The listing builds one solid part. Answer for the finished solid, in the listing's coordinates (mm). A direction names the side the tool comes from. Coordinates: 2 decimals unless noted, no trailing zeros. Order: outer loops, then holes, each group sorted by start corner. A loop starts at its lowest first (then second) coordinate and runs counter-clockwise, first axis right, second up. Notation, with made-up numbers: (-27, 45) - (-20, 45) arc R16 ccw to (-20, 72) - close; hole circle Ø10 at (76, 63.5). An arc over 180 degrees is marked (long way). Use a Markdown table: item, result. Add a question column.
Item 1: Flat-ended cylindrical pins translate along their axes: P1, Ø2, axis at x = -5.5, y = 15, coming from the +Z side; P2, Ø9, axis at x = -1, z = -9, coming from the +Y side; P3, Ø2.5, axis at x = -2, y = 14, coming from the +Z side. Find the tip coordinate at first contact, or state that the pin passes through.
Item 2: The part is cut by section D-D, the plane x = 6.25. Give the vertices of the cut face in (y, z), then the cut area to 3 significant figures.
Item 3: The mould has two halves that part along X. Classify faces 5 (the cylindrical face through (0.358, 17.477, -26.105)), 6 (the flat face through (0, 4, 0)), 7 (the cylindrical face through (0.596, 3.882, -4.815)), 8 (the flat face through (-6, 12.1, -28.2)): released by +X, released by -X, zero draft, split by the parting line, or undercut.
Item 4: The part is cut by section A-A, the plane x = 0. Give the vertices of the cut face in (y, z) (3 decimals).
Item 5: For faces 1 (the flat face through (0.9, 7.9, -10.4)), 2 (the flat face through (-6.1, 1.9, -7.6)), 3 (the flat face through (-6, 4, -15.5)), 4 (the flat face through (-6, 5.75, -8)), determine the directions among +Z, -Z, +X, -X, +Y, -Y from which every point of the face is accessible in a straight line to the end or side of a thin tool.
Item 6: Find the intervals of material crossed by line 1 along Z through (x, y) = (0, 3.5); line 2 along Y through (x, z) = (-6, -27.75); line 3 along Z through (x, y) = (-2.5, 18), in increasing order.
Item 7: The part is cut by section B-B, the plane y = 14.75. Give the vertices of the cut face in (x, z).
Item 8: The part is cut by section C-C, the plane z = -7.5. Give the vertices of the cut face in (x, y) (3 decimals).
from build123d import *

# Parameters (mm, degrees)
ESTRUSIONE_ESTRUSIONE1_DEPTH   = 15.5
SCHIZZO2_W                     = 8
SCHIZZO2_H                     = 7.9
ESTRUSIONE_ESTRUSIONE2_DEPTH   = 14.5
ESTRUSIONE_ESTRUSIONE3_DEPTH   = 18
RACCORDO1_R                    = 1
FORO_PER_VITE_M5_1_D           = 5.5
FORO_PER_VITE_M5_1_DEPTH       = 7.9
FORO_PER_VITE_M5_1_CSINK_D     = 5.55
FORO_PER_VITE_M5_1_CSINK_ANGLE = 90
FORO_PER_VITE_M5_2_D           = 5.5


with BuildPart() as part:
    # Schizzo1 → Estrusione-Estrusione1 (new body)
    with BuildSketch(Plane.XY):
        Polygon((-4.15, 0), (4.15, 0), (8, 3.75), (8, 5.75), (4, 5.75), (4, 7.9), (-4, 7.9), (-4, 5.75), (-8, 5.75), (-8, 3.75), align=None)
    extrude(amount=-ESTRUSIONE_ESTRUSIONE1_DEPTH)

    # Schizzo2 → Estrusione-Estrusione2 (add)
    with BuildSketch(Plane(origin=(0, 0, -15.5), x_dir=(-1, 0, 0), z_dir=(0, 0, -1))):
        with Locations((0, 3.95)):
            Rectangle(SCHIZZO2_W, SCHIZZO2_H)
    extrude(amount=ESTRUSIONE_ESTRUSIONE2_DEPTH)

    # Schizzo4 → Estrusione-Estrusione3 (add)
    with BuildSketch(Plane(origin=(0, 21, 0), x_dir=(-1, 0, 0), z_dir=(0, -1, 0))):
        Polygon((-4.15, 30), (4.15, 30), (8, 26.25), (8, 24.25), (4, 24.25), (4, 22.1), (-4, 22.1), (-4, 24.25), (-8, 24.25), (-8, 26.25), align=None)
    extrude(amount=ESTRUSIONE_ESTRUSIONE3_DEPTH)

    # Raccordo1
    raccordo1_edges = [part.edges().sort_by_distance(p)[0] for p in [
        (0, 7.9, -22.1),
    ]]
    fillet(raccordo1_edges, radius=RACCORDO1_R)

    # Foro per Vite M5-1
    with Locations(Plane(origin=(0, 7.9, 0), x_dir=(1, 0, 0), z_dir=(0, 1, 0))):
        with Locations((0, 7.5)):
            CounterSinkHole(FORO_PER_VITE_M5_1_D / 2, FORO_PER_VITE_M5_1_CSINK_D / 2, depth=FORO_PER_VITE_M5_1_DEPTH, counter_sink_angle=FORO_PER_VITE_M5_1_CSINK_ANGLE)

    # Foro per Vite M5-2 (through all)
    with Locations(Plane.XY.offset(-22.1)):
        with Locations((0, 14.75)):
            Hole(FORO_PER_VITE_M5_2_D / 2)


solid = part.part
Solution:
| question | item | result |
|---|---|---|
| 1 | P1 | stops at z = -24.25 |
| 1 | P2 | stops at y = 7.9 |
| 1 | P3 | stops at z = -22.1 |
| 2 | outline | (2.05, -15.5) - (5.75, -15.5) - (5.75, 0) - (2.05, 0) - close; (3, -27.95) - (21, -27.95) - (21, -24.25) - (3, -24.25) - close |
| 2 | area | 124 mm2 |
| 3 | face 5 | undercut |
| 3 | face 6 | zero draft |
| 3 | face 7 | undercut |
| 3 | face 8 | released by -X |
| 4 | outline | (0, -30) - (12, -30) - (12, -22.1) - (8.9, -22.1) arc R1 cw to (7.9, -21.1) - (7.9, -10.275) - (7.875, -10.25) - (0, -10.25) - close; (0, -4.75) - (7.875, -4.75) - (7.9, -4.725) - (7.9, 0) - (0, 0) - close; (17.5, -30) - (21, -30) - (21, -22.1) - (17.5, -22.1) - close |
| 5 | face 1 | +Z, +X, -X, +Y |
| 5 | face 2 | +Z, -X, -Y |
| 5 | face 3 | -X, +Y, -Y |
| 5 | face 4 | +Z, -X, +Y |
| 6 | line 1 | z = -30 to -10.25, -4.75 to 0 |
| 6 | line 2 | y = 3 to 21 |
| 6 | line 3 | z = -30 to -22.1 |
| 7 | outline | (-8, -26.25) - (-4.15, -30) - (-2.75, -30) - (-2.75, -22.1) - (-4, -22.1) - (-4, -24.25) - (-8, -24.25) - close; (2.75, -30) - (4.15, -30) - (8, -26.25) - (8, -24.25) - (4, -24.25) - (4, -22.1) - (2.75, -22.1) - close |
| 8 | outline | (-8, 3.75) - (-4.15, 0) - (-2.75, 0) - (-2.75, 7.875) - (-2.775, 7.9) - (-4, 7.9) - (-4, 5.75) - (-8, 5.75) - close; (2.75, 0) - (4.15, 0) - (8, 3.75) - (8, 5.75) - (4, 5.75) - (4, 7.9) - (2.775, 7.9) - (2.75, 7.875) - close |
